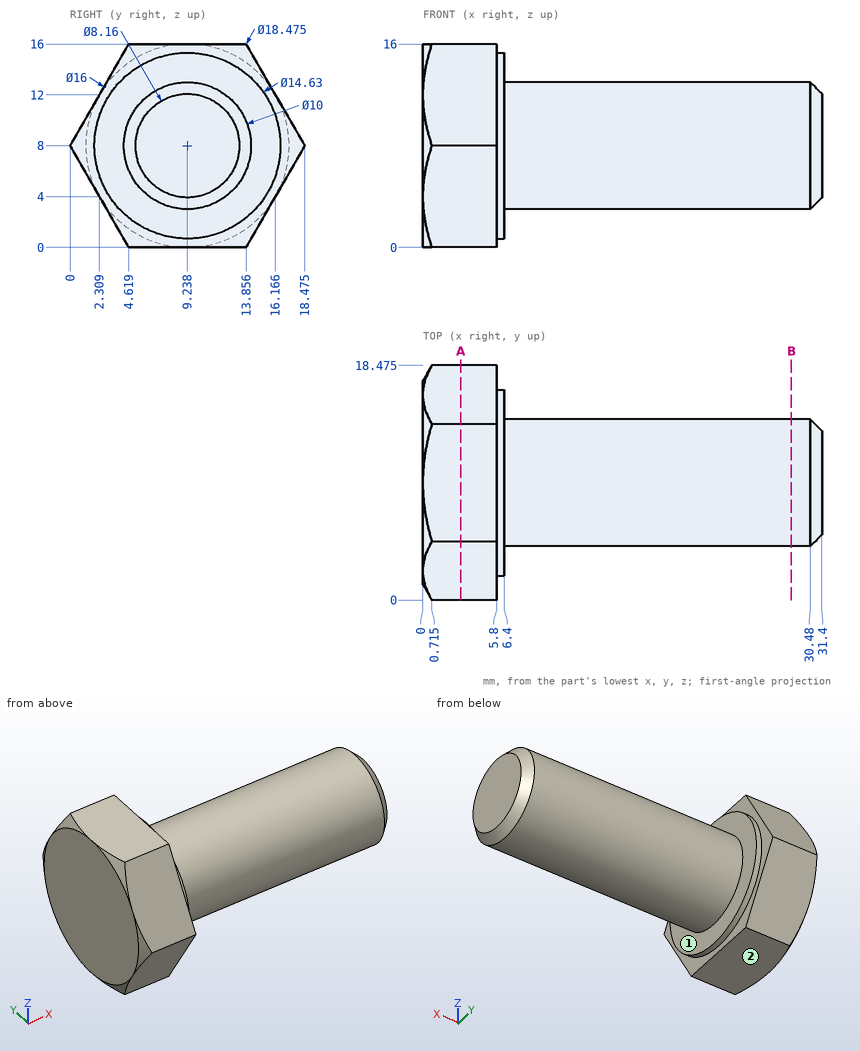
Job drawing, mm, ordinate dimensions from the low corner. One solid piece. A direction names the side the tool comes from. Give positions to 0.01 mm unless a question says otherwise; leave off trailing zeros. Order: outer loops, then holes, each group sorted by start corner. A loop starts at its lowest first (then second) coordinate and runs counter-clockwise, first axis right, second up. Notation, with made-up numbers: M 46.5,59 L 72.5,59 A14 ccw 72.5,80 Z; hole C -29,-12 d7. An arc over 180 degrees is marked long. Return JSON: item names as keys, results as strings.
Q1. Band-saw the part on B-B (x = 29). Give the cut face in (y, z).
Answer list:
{"outline": "C 9.24,8 d10"}
Q2. Wall check: probe 1 along X at (y, z) = (3, 9.75); probe 2 along X at (y, z) = (14.25, 1.75) (1 decimal); probe 3 along Y at (x, z) = (9, 6) (1 decimal). Give the ranges that are in metal, low to high. Write a range as from..to.
Answer list:
{"probe 1": "x = 0..6.4", "probe 2": "x = 0..5.8", "probe 3": "y = 4.7..13.8"}
Q3. 3-axis set-ups, long thin cutter, end or side, ignore diameter. For the marked faces 1 and 2: which of +Z, -Z, +X, -X, +Y, -Y reach the whole face in a straight line?
Answer list:
{"face 1": "+X", "face 2": "-Z, +X, -X, +Y, -Y"}
Q4. Flat gauge pins, fed straight in: pin 1 (5 mm diameter, centred on x = 20.5, y = 16, fed in from +Z) (1 decimal); pin 2 (3 mm diameter, centred on y = 3.5, z = 14, fed in from +X); pin 3 (1 mm diameter, centred on x = 3.5, y = 15.5, fed in from +Z). Where does each tip first touch, or does it go through?
Answer list:
{"pin 1": "stops at z = 10.6", "pin 2": "stops at x = 6.4", "pin 3": "stops at z = 14.02"}
Q5. Band-saw the part on A-A (x = 3). Give the cut face in (y, z) (1 decimal), then the cut area to 3 significant figures.
Answer list:
{"outline": "M 0,8 L 4.6,0 L 13.9,0 L 18.5,8 L 13.9,16 L 4.6,16 Z", "area": "222 mm^2"}
